Autodesk Inventor part; units mm, degrees
ref_plane "YZ Plane" through (0, 0, 0) normal (1, 0, 0) x (0, 1, 0)
ref_plane "XZ Plane" through (0, 0, 0) normal (0, 1, 0) x (-1, 0, 0)
ref_plane "XY Plane" through (0, 0, 0) normal (0, 0, 1) x (1, 0, 0)
sketch "스케치1" plane through (0, 0, 0) normal (0, 0, 1) x (1, 0, 0)
  circle A0 centre (0, 0) radius 21.2
  line L0 (25, -22.5) -> (25, 27.5)
  line L1 (-25, 27.5) -> (-25, -22.5)
  circle A1 centre (0, 0) radius 22.3
  line L2 (25, 27.5) -> (-25, 27.5)
  line L3 (-11.7, 4.9396) -> (-11.7, -4.9396)
  arc A2 (-11.7, -4.9396) -> (11.7, -4.9396) centre (0, 0) ccw
  line L4 (11.7, -4.9396) -> (11.7, 4.9396)
  arc A3 (11.7, 4.9396) -> (-11.7, 4.9396) centre (0, 0) ccw
  circle A4 centre (12.3744, -12.3744) radius 2.1
  circle A5 centre (12.3744, 12.3744) radius 2.1
  circle A6 centre (-12.3744, 12.3744) radius 2.1
  circle A7 centre (-12.3744, -12.3744) radius 2.1
  line L5 (50, -22.5) -> (-50, -22.5)
  line L6 (50, -22.5) -> (50, -2.5)
  line L7 (50, -2.5) -> (25, 27.5)
  line L8 (-50, -22.5) -> (-50, -2.5)
  line L9 (-50, -2.5) -> (-25, 27.5)
  line L10 (-50, -22.5) -> (-65, -22.5)
  line L11 (50, -22.5) -> (65, -22.5)
  line L12 (65, -22.5) -> (65, -2.5)
  line L13 (-65, -22.5) -> (-65, -2.5)
  line L14 (-65, -2.5) -> (-25, 27.5)
  line L15 (25, 27.5) -> (65, -2.5)
  line L16 (-65, -22.5) -> (-65, 7.5)
  line L17 (65, -22.5) -> (65, 7.5)
  line L18 (25, -22.5) -> (25, 37.5)
  line L19 (-25, -22.5) -> (-25, 37.5)
  line L20 (-25, 37.5) -> (-65, 7.5)
  line L21 (-25, 37.5) -> (25, 37.5)
  line L22 (25, 37.5) -> (65, 7.5)
  line L23 (-25, 37.5) -> (-35, 37.5)
  line L24 (-35, 37.5) -> (-65, 7.5)
  line L25 (25, 37.5) -> (35, 37.5)
  line L26 (35, 37.5) -> (65, 7.5)
  dimension "d17" = 360
  dimension "d29" = 20
  dimension "d30" = 20
  dimension "d33" = 15
  dimension "d34" = 15
  dimension "d35" = 30
  dimension "d36" = 30
  dimension "d37" = 60
  dimension "d38" = 60
  dimension "d39" = 10
  dimension "d40" = 10
extrude "판1" add sketch "스케치1" along normal blind 5 contours A0 | L5 L1 L2 L0 | L0 L7 L6 L5 | L15 L12 L11 L6 L7 | L18 L22 L17 L15 | L2 L19 L21 L18 | L5 L8 L9 L1 | L9 L8 L10 L13 L14 | L14 L16 L20 L19 | L25 L26 L22 | L20 L24 L23 | A1
fillet "모서리 라운드2" radius 6 4 edges at (-35, 37.5, 2.5) (-65, 7.5, 2.5) (35, 37.5, 2.5) (65, 7.5, 2.5)
sketch "스케치2" plane through (0, 0, 5) normal (0, 0, 1) x (1, 0, 0)
  line L0 (-65, -22.5) -> (-65, 5.0147)
  line L1 (-65, -22.5) -> (-60, -22.5)
  line L2 (65, -22.5) -> (-65, -22.5)
  line L3 (65, -22.5) -> (60, -22.5)
  line L4 (60, -22.5) -> (30, -22.5)
  line L5 (30, -22.5) -> (30, 7.5)
  line L6 (30, 7.5) -> (60, 7.5)
  line L7 (60, 7.5) -> (60, -22.5)
  line L8 (-60, -22.5) -> (-30, -22.5)
  line L9 (-30, -22.5) -> (-30, 7.5)
  line L10 (-30, 7.5) -> (-60, 7.5)
  line L11 (-60, 7.5) -> (-60, -22.5)
  line L12 (-60, -22.5) -> (-45, -22.5)
  line L13 (-45, -22.5) -> (-45, -7.5)
  line L14 (60, -22.5) -> (45, -22.5)
  line L15 (45, -22.5) -> (45, -7.5)
  circle A0 centre (45, -7.5) radius 2.6
  circle A1 centre (-45, -7.5) radius 2.6
  point P0 (0, 0)
  dimension "d42" = 5
  dimension "d43" = 5
  dimension "d44" = 30
  dimension "d45" = 30
  dimension "d46" = 30
  dimension "d47" = 30
  dimension "d48" = 15
  dimension "d49" = 5.2
  dimension "d50" = 5.2
extrude "돌출1" cut sketch "스케치2" against normal through all contours A0 | A1
sketch "스케치3" plane through (0, 0, 5) normal (0, 0, 1) x (1, 0, 0)
  line L0 (65, -22.5) -> (-65, -22.5)
  line L1 (-65, -22.5) -> (65, -22.5)
  line L2 (65, -22.5) -> (65, -27.5)
  line L3 (65, -27.5) -> (-65, -27.5)
  line L4 (-65, -27.5) -> (-65, -22.5)
  line L5 (-65, -22.5) -> (-39, -22.5)
  line L6 (-39, -22.5) -> (-13, -22.5)
  line L7 (-13, -22.5) -> (13, -22.5)
  line L8 (13, -22.5) -> (39, -22.5)
  line L9 (39, -22.5) -> (65, -22.5)
  line L10 (-39, -22.5) -> (-39, -27.5)
  line L11 (-13, -22.5) -> (-13, -27.5)
  line L12 (13, -22.5) -> (13, -27.5)
  line L13 (39, -22.5) -> (39, -27.5)
  point P0 (0, 0)
  dimension "d53" = 130
  dimension "d54" = 5
  dimension "d55" = 26
  dimension "d56" = 26
  dimension "d57" = 26
  dimension "d58" = 26
  dimension "d59" = 26
extrude "돌출2" add sketch "스케치3" against normal blind 5 contours L2 L3 L13 L0 | L12 L3 L11 L0 | L10 L3 L4 L0
equation "\"TransitionRadius\" = BendRadius"
properties part number "motor_wall" material "알루미늄 6061"
Here's how the part is built. I have some questions about the finished solid (model axes, mm). A direction names the side the tool comes from. Round coordinates to 2 decimals unless told otherwise and drop trailing zeros. Write each loop counter-clockwise with the first axis right and the second up, starting at its lowest first coordinate (ties: lowest second). Pieces come first, ordered by that corner, then holes.
1. For faces 1 (the flat face through (11.7, 0, 2)), 2 (the flat face through (65, -11, 2)), 3 (the flat face through (-13, -25, 3)), which set-ups out of +Z, -Z, +X, -X, +Y, -Y let a thin tool reach every point of the face, with its end or its side?
2. Suppose I cut it at B-B (y = -7.5). List the corners of the cut face in (x, z) for me, and give its area (3 significant figures).
3. Suppose I cut it at A-A (x = -45). List the corners of the cut face in (y, z) for me, and give its area (3 significant figures).
4. Suppose I cut it at C-C (z = 4). List the corners of the cut face in (x, y) for me.
5. Suppose I cut it at D-D (x = 28). List the corners of the cut face in (y, z) for me.
6. Will this pin go through, and if not, where does the flat tip stop? pin 1 Ø2.5 at (x, z) = (-30, 2) entering from -Y.
7. I need wall thicknesses on L1, parallel to X at y = 0, z = 3.95; L2, parallel to X at y = 13, z = 2; L3, parallel to Y at x = 12, z = 3.1. Which ranges of each line are inside material? Lowest first, please.
8. If we mould it in two halves opening along Y, with no side actions, what happens to faces 4 (the flat face through (-1, 13, 5)), 5 (the flat face through (49.8, 22.7, 2.5)), 6 (the cylindrical face through (11.919, 14.424, 2.465))? For each: released by +Y, released by -Y, zero draft, split by the parting line, or undercut.
Answer sheet:
1. face 1: +Z, -Z
1. face 2: +Z, -Z, +X, +Y, -Y
1. face 3: +Z, -Z, -Y
2. outline: (-65, 0) - (-47.6, 0) - (-47.6, 5) - (-65, 5) - close; (-42.4, 0) - (-10.25, 0) - (-10.25, 5) - (-42.4, 5) - close; (10.25, 0) - (42.4, 0) - (42.4, 5) - (10.25, 5) - close; (47.6, 0) - (65, 0) - (65, 5) - (47.6, 5) - close
2. area: 496 mm2
3. outline: (-27.5, 0) - (-10.1, 0) - (-10.1, 5) - (-27.5, 5) - close; (-4.9, 0) - (27.5, 0) - (27.5, 5) - (-4.9, 5) - close
3. area: 249 mm2
4. outline: (-65, -27.5) - (-39, -27.5) - (-39, -22.5) - (-13, -22.5) - (-13, -27.5) - (13, -27.5) - (13, -22.5) - (39, -22.5) - (39, -27.5) - (65, -27.5) - (65, 5.01) arc R6 ccw to (63.24, 9.26) - (36.76, 35.74) arc R6 ccw to (32.51, 37.5) - (-32.51, 37.5) arc R6 ccw to (-36.76, 35.74) - (-63.24, 9.26) arc R6 ccw to (-65, 5.01) - close; hole circle Ø5.2 at (-45, -7.5); hole circle Ø4.2 at (-12.37, -12.37); hole circle Ø4.2 at (-12.37, 12.37); hole (-11.7, -4.94) arc R12.7 ccw to (11.7, -4.94) - (11.7, 4.94) arc R12.7 ccw to (-11.7, 4.94) - close; hole circle Ø4.2 at (12.37, -12.37); hole circle Ø4.2 at (12.37, 12.37); hole circle Ø5.2 at (45, -7.5)
5. outline: (-22.5, 0) - (37.5, 0) - (37.5, 5) - (-22.5, 5) - close
6. pin 1: stops at y = -22.5
7. L1: x = -65 to -11.7, 11.7 to 65
7. L2: x = -59.5 to -14.38, -10.37 to 10.37, 14.38 to 59.5
7. L3: y = -27.5 to -14.44, -10.31 to 10.31, 14.44 to 37.5
8. face 4: zero draft
8. face 5: released by +Y
8. face 6: undercut
